```python
from build123d import *

# Parameters (mm, degrees)
F1_DEPTH  = 10
F2_R      = 1.5
F3_DEPTH  = 15
F4_R      = 1.5
F5_DEPTH  = 0.5
F6_R      = 1.5
F7_DEPTH  = 0.5
F8_W      = 1
F8_H      = 6
F9_DEPTH  = 10
F10_W     = 1
F10_H     = 6.5
F11_DEPTH = 3.5
F12_W     = 1
F12_H     = 6.5
F13_DEPTH = 10
F14_W     = 1
F14_H     = 4
F15_DEPTH = 2
F16_W     = 1
F16_H     = 4
F17_DEPTH = 51


with BuildPart() as f1:
    # F0 (on Top) → F1 (new body)
    with BuildSketch(Plane.XY):
        with BuildLine():
            Line((11.152231, 4.569918), (-11.847769, 4.569918))
            ThreePointArc((-11.847769, 4.569918), (-13.615536, 3.837685), (-14.347769, 2.069918))
            Line((-14.347769, 2.069918), (-14.347769, -7.930082))
            ThreePointArc((-14.347769, -7.930082), (-13.615536, -9.697848), (-11.847769, -10.430082))
            Line((-11.847769, -10.430082), (11.152231, -10.430082))
            ThreePointArc((11.152231, -10.430082), (12.919998, -9.697848), (13.652231, -7.930082))
            Line((13.652231, -7.930082), (13.652231, 2.069918))
            ThreePointArc((13.652231, 2.069918), (12.919998, 3.837685), (11.152231, 4.569918))
        make_face()
    extrude(amount=F1_DEPTH)

    # F2 (on face) → F3 (cut)
    with BuildSketch(Plane.XY.offset(10)):
        with Locations((-11.847769, 2.069918)):
            Circle(F2_R)
        with Locations((11.152231, -7.930082)):
            Circle(F2_R)
    extrude(amount=-F3_DEPTH, mode=Mode.SUBTRACT)

    # F4 (on face) → F5 (join)
    with BuildSketch(Plane.XY.offset(10)):
        with BuildLine():
            Line((-9.347769, 1.069918), (-9.347769, 4.569918))
            Line((-9.347769, 4.569918), (-11.847769, 4.569918))
            ThreePointArc((-11.847769, 4.569918), (-13.615536, 3.837685), (-14.347769, 2.069918))
            Line((-14.347769, 2.069918), (-14.347769, 0.069918))
            Line((-14.347769, 0.069918), (-10.347769, 0.069918))
            ThreePointArc((-10.347769, 0.069918), (-9.640663, 0.362812), (-9.347769, 1.069918))
        make_face()
        with Locations((-11.847769, 2.069918)):
            Circle(F4_R, mode=Mode.SUBTRACT)
        with BuildLine():
            Line((13.652231, -7.930082), (13.652231, -5.930082))
            Line((13.652231, -5.930082), (9.652231, -5.930082))
            ThreePointArc((9.652231, -5.930082), (8.945124, -6.222975), (8.652231, -6.930082))
            Line((8.652231, -6.930082), (8.652231, -10.430082))
            Line((8.652231, -10.430082), (11.152231, -10.430082))
            ThreePointArc((11.152231, -10.430082), (12.919998, -9.697848), (13.652231, -7.930082))
        make_face()
        with Locations((11.152231, -7.930082)):
            Circle(F4_R, mode=Mode.SUBTRACT)
    extrude(amount=F5_DEPTH)

    # F6 (on face) → F7 (join)
    with BuildSketch(Plane(origin=(0, 0, 0), x_dir=(1, 0, 0), z_dir=(0, 0, -1))):
        with BuildLine():
            Line((-10.347769, -0.069918), (-14.347769, -0.069918))
            Line((-14.347769, -0.069918), (-14.347769, -2.069918))
            ThreePointArc((-14.347769, -2.069918), (-13.615536, -3.837685), (-11.847769, -4.569918))
            Line((-11.847769, -4.569918), (-9.347769, -4.569918))
            Line((-9.347769, -4.569918), (-9.347769, -1.069918))
            ThreePointArc((-9.347769, -1.069918), (-9.640663, -0.362812), (-10.347769, -0.069918))
        make_face()
        with Locations((-11.847769, -2.069918)):
            Circle(F6_R, mode=Mode.SUBTRACT)
        with BuildLine():
            Line((11.152231, 10.430082), (8.652231, 10.430082))
            Line((8.652231, 10.430082), (8.652231, 6.930082))
            ThreePointArc((8.652231, 6.930082), (8.945124, 6.222975), (9.652231, 5.930082))
            Line((9.652231, 5.930082), (13.652231, 5.930082))
            Line((13.652231, 5.930082), (13.652231, 7.930082))
            ThreePointArc((13.652231, 7.930082), (12.919998, 9.697848), (11.152231, 10.430082))
        make_face()
        with Locations((11.152231, 7.930082)):
            Circle(F6_R, mode=Mode.SUBTRACT)
    extrude(amount=F7_DEPTH)

    # F8 (on face) → F9 (join)
    with BuildSketch(Plane.YZ.offset(13.652231)):
        with Locations((-6.430082, 5)):
            Rectangle(F8_W, F8_H)
    extrude(amount=F9_DEPTH)

    # F10 (on face) → F11 (join)
    with BuildSketch(Plane.XZ.offset(10.430082)):
        with Locations((1.152231, 5)):
            Rectangle(F10_W, F10_H)
    extrude(amount=F11_DEPTH)

    # F12 (on face) → F13 (join)
    with BuildSketch(Plane.YZ.offset(1.652231)):
        with Locations((-13.430082, 5)):
            Rectangle(F12_W, F12_H)
    extrude(amount=F13_DEPTH)

    # F14 (on face) → F15 (join)
    with BuildSketch(Plane(origin=(0, 4.569918, 0), x_dir=(-1, 0, 0), z_dir=(0, 1, 0))):
        with Locations((3.347769, 5)):
            Rectangle(F14_W, F14_H)
    extrude(amount=F15_DEPTH)

    # F16 (on face) → F17 (join)
    with BuildSketch(Plane(origin=(-3.847769, 0, 0), x_dir=(0, -1, 0), z_dir=(-1, 0, 0))):
        with Locations((-6.069918, 5)):
            Rectangle(F16_W, F16_H)
    extrude(amount=F17_DEPTH)


solid = f1.part
```
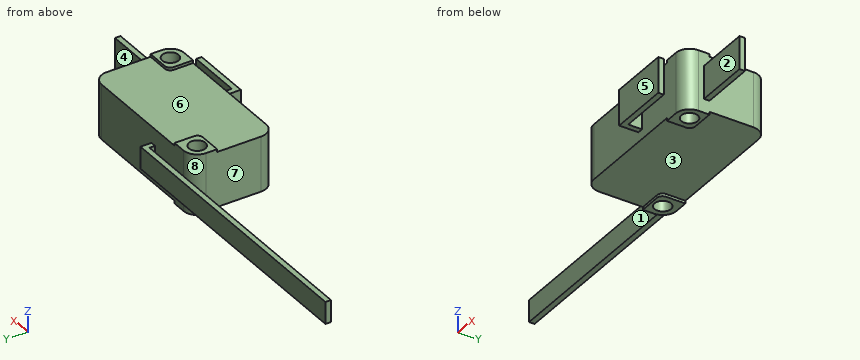
Model file for the job. Use its own axes, mm. Face numbers are marked on the shaded views. A direction names the side the tool comes from. Coordinates: 2 decimals unless noted, no trailing zeros. Write each loop counter-clockwise with the first axis right and the second up, starting at its lowest first coordinate (ties: lowest second). Pieces come first, ordered by that corner, then holes. Notation, with made-up numbers: (55.25, -37.75) - (77.25, -37.75) arc R29 cw to (77.25, -4.75) - close; hole circle Ø5 at (-8, 53). An arc over 180 degrees is marked (long way). Use a Markdown table: item, result. Add a question column.
Item 1: Band-saw the part on B-B, the plane y = -2. Write the cut outline in (x, z), and give its area (3 significant figures).
Item 2: Drop flat-ended pins along their axis: pin 1 (12 mm diameter, centred on x = 1, y = -5, fed in from +Z); pin 2 (1.8 mm diameter, centred on x = 18.5, z = 6, fed in from +Y); pin 3 (1 mm diameter, centred on x = -25.5, y = 5.5, fed in from +Z); pin 4 (1.8 mm diameter, centred on x = -11.85, y = 2.07, fed in from +Z). Give the stop position or say it passes through.
Item 3: Band-saw the part on A-A, the plane z = 1. Write the cut outline in (x, y).
Item 4: Two-plate mould, pull along Y, no slides. Class the marked faces 1, 2 and 3: pulls with the +Y half, pulls with the -Y half, needs draft (parallel to the pull), parting line crosses it, or undercut.
Item 5: 3-axis set-ups, long thin cutter, end or side, ignore diameter. For the marked faces 4, 5, 6, 7 and 8: which of +Z, -Z, +X, -X, +Y, -Y reach the whole face in a straight line?
Item 6: Band-saw the part on C-C, the plane x = -29. Write the cut outline in (y, z), and give its area (3 significant figures).
Item 7: Band-saw the part on D-D, the plane z = 5.75. Write the cut outline in (x, y).
Item 8: Drill centre lines: line 1 along Y through (x, z) = (6.5, 5); line 2 along Y through (x, z) = (-6, 3.25); line 3 along Y through (x, z) = (-13, 3.5). Where is each one in solid material? Low to high.
A:
| question | item | result |
|---|---|---|
| 1 | outline | (-14.35, 0) - (13.65, 0) - (13.65, 10) - (-14.35, 10) - close |
| 1 | area | 280 mm² |
| 2 | pin 1 | stops at z = 10 |
| 2 | pin 2 | stops at y = -5.93 |
| 2 | pin 3 | stops at z = 7 |
| 2 | pin 4 | passes through |
| 3 | outline | (-14.35, -7.93) arc R2.5 ccw to (-11.85, -10.43) - (11.15, -10.43) arc R2.5 ccw to (13.65, -7.93) - (13.65, 2.07) arc R2.5 ccw to (11.15, 4.57) - (-11.85, 4.57) arc R2.5 ccw to (-14.35, 2.07) - close; hole circle Ø3 at (-11.85, 2.07); hole circle Ø3 at (11.15, -7.93) |
| 4 | face 1 | undercut |
| 4 | face 2 | pulls with the -Y half |
| 4 | face 3 | needs draft |
| 5 | face 4 | +Z, -Z, +X, +Y |
| 5 | face 5 | +Z, -Z, +X, -X, -Y |
| 5 | face 6 | +Z |
| 5 | face 7 | +Z, -Z, -X, -Y |
| 5 | face 8 | +Z, -Z, -X |
| 6 | outline | (5.57, 3) - (6.57, 3) - (6.57, 7) - (5.57, 7) - close |
| 6 | area | 4.00 mm² |
| 7 | outline | (-54.85, 5.57) - (-3.85, 5.57) - (-3.85, 4.57) - (-11.85, 4.57) arc R2.5 ccw to (-14.35, 2.07) - (-14.35, -7.93) arc R2.5 ccw to (-11.85, -10.43) - (0.65, -10.43) - (0.65, -13.93) - (11.65, -13.93) - (11.65, -12.93) - (1.65, -12.93) - (1.65, -10.43) - (11.15, -10.43) arc R2.5 ccw to (13.65, -7.93) - (13.65, -6.93) - (23.65, -6.93) - (23.65, -5.93) - (13.65, -5.93) - (13.65, 2.07) arc R2.5 ccw to (11.15, 4.57) - (-2.85, 4.57) - (-2.85, 6.57) - (-54.85, 6.57) - close; hole circle Ø3 at (-11.85, 2.07); hole circle Ø3 at (11.15, -7.93) |
| 8 | line 1 | y = -13.93 to -12.93, -10.43 to 4.57 |
| 8 | line 2 | y = -10.43 to 4.57, 5.57 to 6.57 |
| 8 | line 3 | y = -10.15 to 1.11, 3.03 to 4.29, 5.57 to 6.57 |
